The drawing under review shows one solid part. Ordinate dimensions are in mm from its lowest x, y, z. Round coordinates to 2 decimals unless told otherwise and drop trailing zeros. Order: outer loops, then holes, each group sorted by start corner. A loop starts at its lowest first (then second) coordinate and runs counter-clockwise, first axis right, second up. Notation, with made-up numbers: (9.25, 78) -> (18.25, 78) arc R26 cw to (18.25, 95) -> close; hole circle Ø1 at (-23, -1). An arc over 180 degrees is marked (long way). Use a Markdown table: item, result. Add a question column.
1) Consider section A-A (z = 2.1). State the section outline as (x, y) points, plus the area to 3 significant figures.
2) Consider section C-C (y = 17.25). State the section outline as (x, z) points.
3) Draft analysis for pull direction Y (two halves, no side actions). For the marked faces 1, 2 and 3, state which applies: pulls with the +Y half, pulls with the -Y half, needs draft (parallel to the pull), parting line crosses it, or undercut.
4) Clearance check with a flat-ended pin moving along its axis: P1, Ø5.5, axis at x = 7.5, y = 11.5, coming from the +Z side. State where the tip first meets the part, or that it passes through.
5) Consider section B-B (x = 24.25). State the section outline as (y, z) points, plus the area to 3 significant figures.
6) Wall thickness on line 1 along Y through (x, z) = (12.5, 1.25); line 2 along X through (y, z) = (17.75, 2.05); line 3 along Z through (x, y) = (7, 8.5): over which ranges is each line inside the solid? List them lowest first. Write a range as [from, to].
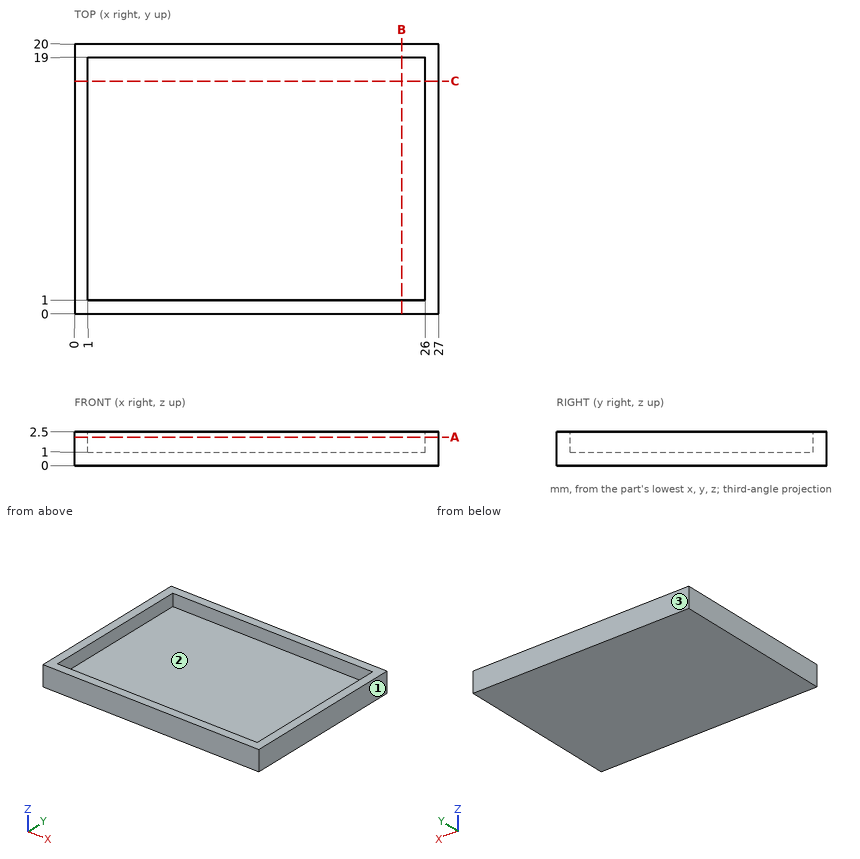
Results list:
| question | item | result |
|---|---|---|
| 1 | outline | (0, 0) -> (27, 0) -> (27, 20) -> (0, 20) -> close; hole (1, 1) -> (26, 1) -> (26, 19) -> (1, 19) -> close |
| 1 | area | 90.0 mm2 |
| 2 | outline | (0, 0) -> (27, 0) -> (27, 2.5) -> (26, 2.5) -> (26, 1) -> (1, 1) -> (1, 2.5) -> (0, 2.5) -> close |
| 3 | face 1 | needs draft |
| 3 | face 2 | undercut |
| 3 | face 3 | pulls with the +Y half |
| 4 | P1 | z = 1 |
| 5 | outline | (0, 0) -> (20, 0) -> (20, 2.5) -> (19, 2.5) -> (19, 1) -> (1, 1) -> (1, 2.5) -> (0, 2.5) -> close |
| 5 | area | 23.0 mm2 |
| 6 | line 1 | [0, 1], [19, 20] |
| 6 | line 2 | [0, 1], [26, 27] |
| 6 | line 3 | [0, 1] |
